The listing builds one solid part. Answer for the finished solid, in the listing's coordinates (mm). Face numbers are marked on the shaded views. A direction names the side the tool comes from. Coordinates: 2 decimals unless noted, no trailing zeros. Loops run counter-clockwise (first coordinate to the right, second up) from the corner with the lowest first, then second, coordinate; pieces in that order, holes last. Notation, with made-up numbers: (83.5, 44) - (123.5, 44) arc R8 cw to (123.5, 53) - close; hole circle Ø10 at (14, -20). An arc over 180 degrees is marked (long way). Put each result on its own line as item: value.
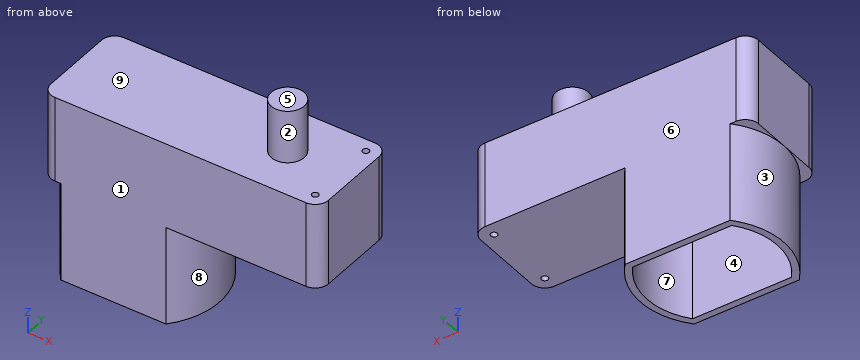
```python
from build123d import *

# Parameters (mm, degrees)
BOSS_EXTRUDE1_DEPTH = 15
SKETCH2_W           = 42
SKETCH2_H           = 15
BOSS_EXTRUDE2_DEPTH = 13
FILLET1_R           = 2
SKETCH3_R           = 2.5
BOSS_EXTRUDE3_DEPTH = 8
SKETCH4_R           = 0.5
CUT_EXTRUDE1_DEPTH  = 43.558628129


with BuildPart() as part:
    # Sketch1 → Boss-Extrude1 (new body)
    with BuildSketch(Plane.XY):
        with BuildLine():
            ThreePointArc((7.957391107, 7.5), (10.83933845, 0), (7.957391107, -7.5))
            Line((7.957391107, -7.5), (-7.957391107, -7.5))
            ThreePointArc((-7.957391107, -7.5), (-10.83933845, 0), (-7.957391107, 7.5))
            Line((-7.957391107, 7.5), (7.957391107, 7.5))
        make_face()
        with BuildLine():
            Line((-7.5, 6.5), (7.5, 6.5))
            ThreePointArc((7.5, 6.5), (9.83933845, 0), (7.5, -6.5))
            Line((7.5, -6.5), (-7.5, -6.5))
            ThreePointArc((-7.5, -6.5), (-9.83933845, 0), (-7.5, 6.5))
        make_face(mode=Mode.SUBTRACT)
    extrude(amount=BOSS_EXTRUDE1_DEPTH)

    # Sketch2 → Boss-Extrude2 (add)
    with BuildSketch(Plane.XY.offset(15)):
        with Locations((10.16066155, 0)):
            Rectangle(SKETCH2_W, SKETCH2_H)
    extrude(amount=BOSS_EXTRUDE2_DEPTH)

    # Fillet1
    fillet1_edges = [part.edges().sort_by_distance(p)[0] for p in [
        (31.16066155, 7.5, 21.5),
        (-10.83933845, 7.5, 21.5),
        (-10.83933845, -7.5, 21.5),
        (31.16066155, -7.5, 21.5),
    ]]
    fillet(fillet1_edges, radius=FILLET1_R)

    # Sketch3 → Boss-Extrude3 (add)
    with BuildSketch(Plane.XY.offset(28)):
        with Locations(Location((21.16066155, 0, 0), (0, 0, 180))):
            Circle(SKETCH3_R)
    extrude(amount=BOSS_EXTRUDE3_DEPTH)

    # Sketch4 → Cut-Extrude1 (cut, through all)
    with BuildSketch(Plane.XY.offset(28)):
        with Locations((29.16066155, 5.5)):
            Circle(SKETCH4_R)
    cut_extrude1 = extrude(amount=-CUT_EXTRUDE1_DEPTH, mode=Mode.SUBTRACT)

    # Mirror1: Cut-Extrude1 across plane
    add(cut_extrude1.mirror(Plane.ZX), mode=Mode.SUBTRACT)


solid = part.part
```
1) Straight lines are drawn through the part: L1, parallel to Z at x = -8, y = -4.5; L2, parallel to Z at x = 22, y = 0.5; L3, parallel to Y at x = 29.5, z = 19. For each, find the intervals that lie inside material, in ascending order. Write a range as [from, to].
Found:
L1: z = [15, 28]
L2: z = [15, 36]
L3: y = [-7.47, -5.87], [-5.13, 5.13], [5.87, 7.47]
2) For a pull along Y with two mould halves and no side action, classify the marked faces 6, 7, 8 and 9 as pulls with the +Y half, pulls with the -Y half, needs draft (parallel to the pull), parting line crosses it, or undercut.
Found:
face 6: pulls with the +Y half
face 7: undercut
face 8: parting line crosses it
face 9: needs draft
3) The part is cut by section C-C (y = 1.5). Give the vertices of the cut face in (x, z).
Found:
outline: (-10.84, 15) - (-10.74, 15) - (-10.74, 0) - (-9.73, 0) - (-9.73, 15) - (9.73, 15) - (9.73, 0) - (10.74, 0) - (10.74, 15) - (31.16, 15) - (31.16, 28) - (23.16, 28) - (23.16, 36) - (19.16, 36) - (19.16, 28) - (-10.84, 28) - close
4) The part is cut by section D-D (z = 30). Give the vertices of the cut face in (x, y).
Found:
outline: circle Ø5 at (21.16, 0)
5) For the marked faces 1, 2, 3, 4 and 5, determine the directions among +Z, -Z, +X, -X, +Y, -Y from which every point of the face is accessible in a straight line to the end or side of a thin tool.
Found:
face 1: +Z, -Z, +X, -X, -Y
face 2: +Z
face 3: -Z, -X
face 4: -Z
face 5: +Z, +X, -X, +Y, -Y
6) Each of these flat-tipped pins is pushed along its axis until it touches: pin 1 (1.5 mm diameter, centred on x = -6, y = -5.5, fed in from +Z); pin 2 (3 mm diameter, centred on x = 10, z = 9.5, fed in from +Y); pin 3 (1 mm diameter, centred on y = 2.5, z = 31, fed in from -X). Where does it stop, or does it pass through?
Found:
pin 1: stops at z = 28
pin 2: stops at y = 6.85
pin 3: stops at x = 19.66
7) The part is cut by section B-B (z = 5). Give the vertices of the cut face in (x, y).
Found:
outline: (-7.96, -7.5) - (7.96, -7.5) arc R11.2 ccw to (7.96, 7.5) - (-7.96, 7.5) arc R11.2 ccw to start; hole (-7.5, -6.5) - (7.5, -6.5) arc R10.2 ccw to (7.5, 6.5) - (-7.5, 6.5) arc R10.2 ccw to start
8) The part is cut by section A-A (x = -3). Give the vertices of the cut face in (y, z).
Found:
outline: (-7.5, 0) - (-6.5, 0) - (-6.5, 15) - (6.5, 15) - (6.5, 0) - (7.5, 0) - (7.5, 28) - (-7.5, 28) - close
